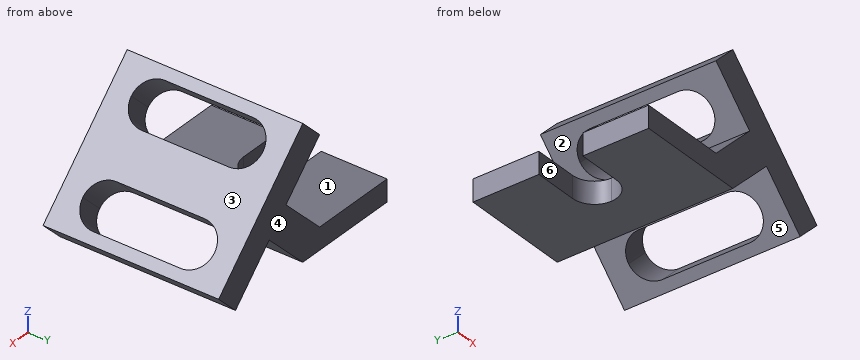
from build123d import *

# Parameters (mm, degrees)
F1_DEPTH = 101.6
F3_DEPTH = 25.4
F5_DEPTH = 37.846


with BuildPart() as f1:
    # F0 (on Front) → F1 (new body, symmetric)
    with BuildSketch(Plane.XZ):
        Polygon((152.4, 76.2), (152.4, 25.4), (177.8, 50.8), (228.6, 0), (254, 25.4), (127, 152.4), (101.6, 127), align=None)
        Polygon((152.4, 76.2), (101.6, 25.4), (152.4, 25.4), align=None)
        Polygon((0, 25.4), (0, 0), (127, 0), (152.4, 25.4), (101.6, 25.4), align=None)
    extrude(amount=F1_DEPTH, both=True)

    # F2 (on face) → F3 (cut)
    with BuildSketch(Plane(origin=(0, 0, 0), x_dir=(1, 0, 0), z_dir=(0, 0, -1))):
        with BuildLine():
            Line((0, 25.4), (0, 0))
            Line((0, 0), (0, -25.4))
            Line((0, -25.4), (50.8, -25.4))
            ThreePointArc((50.8, -25.4), (68.760512, -17.960512), (76.2, 0))
            ThreePointArc((76.2, 0), (68.760512, 17.960512), (50.8, 25.4))
            Line((50.8, 25.4), (0, 25.4))
        make_face()
    extrude(amount=-F3_DEPTH, mode=Mode.SUBTRACT)

    # F4 (on face) → F5 (cut)
    with BuildSketch(Plane(origin=(139.7, 0, 139.7), x_dir=(0, 1, 0), z_dir=(0.707107, 0, 0.707107))):
        with BuildLine():
            ThreePointArc((-76.2, -20.139488), (-68.760512, -38.1), (-50.8, -45.539488))
            Line((-50.8, -45.539488), (50.8, -45.539488))
            ThreePointArc((50.8, -45.539488), (68.760512, -38.1), (76.2, -20.139488))
            ThreePointArc((76.2, -20.139488), (68.760512, -2.178976), (50.8, 5.260512))
            Line((50.8, 5.260512), (-50.8, 5.260512))
            ThreePointArc((-50.8, 5.260512), (-68.760512, -2.178976), (-76.2, -20.139488))
        make_face()
        with BuildLine():
            ThreePointArc((50.8, -148.94461), (68.760512, -141.505122), (76.2, -123.54461))
            ThreePointArc((76.2, -123.54461), (68.760512, -105.584098), (50.8, -98.14461))
            Line((50.8, -98.14461), (-50.8, -98.14461))
            ThreePointArc((-50.8, -98.14461), (-68.760512, -105.584098), (-76.2, -123.54461))
            ThreePointArc((-76.2, -123.54461), (-68.760512, -141.505122), (-50.8, -148.94461))
            Line((-50.8, -148.94461), (50.8, -148.94461))
        make_face()
    extrude(amount=-F5_DEPTH, mode=Mode.SUBTRACT)


solid = f1.part
The model under review builds one solid part; all positions refer to its coordinate system, in mm. Face numbers are marked on the shaded views. A direction names the side the tool comes from. Give positions to 0.01 mm unless a question says otherwise; leave off trailing zeros. Loops run counter-clockwise (first coordinate to the right, second up) from the corner with the lowest first, then second, coordinate; pieces in that order, holes last. Notation, with made-up numbers: (51.25, -17.5) -> (94.25, -17.5) arc R34 cw to (94.25, 21.5) -> close; hole circle Ø3 at (77.5, -15). An arc over 180 degrees is marked (long way). Put each result on its own line as item: value. Start each with the question number.
1. We need section B-B on y = 45. State the section outline as (x, z) points, then the cut area to 3 significant figures.
2. Clearance check with flat-ended pins moving along their axes: P1, Ø3, axis at y = -3.5, z = 118.5, coming from the +X side; P2, Ø10, axis at y = -5, z = 119.5, coming from the -X side; P3, Ø5, axis at y = 5.5, z = 90, coming from the -X side. State where each tip first meets the part, or that it passes through.
3. We need section D-D on y = 3. State the section outline as (x, z) points, then the cut area to 3 significant figures.
4. Wall thickness on probe 1 along Y at (x, z) = (150, 121); probe 2 along Z at (x, y) = (126, 52); probe 3 along Z at (x, y) = (19, 48): over which ranges is each line inside the solid? List them lowest first.
5. Mouldability with a two-part tool opening along Y and no side actions: class the marked faces 4, 5 and 6 as released by +Y, released by -Y, zero draft, split by the parting line, or undercut.
6. We need section C-C on x = 65. State the section outline as (y, z) points, then the cut area to 3 significant figures.
7. We need section A-A on x = 37. State the section outline as (y, z) points, then the cut area to 3 significant figures.
8. For the marked faces 1, 2 and 3, list the 3-axis set-ups (+Z, -Z, +X, -X, +Y, -Y) from which the entire face can be reached by the end or side of a thin tool; tool diameter is ignored.
Determined:
1. outline: (0, 0) -> (127, 0) -> (177.8, 50.8) -> (183.7, 44.9) -> (209.1, 70.3) -> (171.9, 107.5) -> (146.5, 82.1) -> (152.4, 76.2) -> (101.6, 25.4) -> (0, 25.4) -> close; (101.6, 127) -> (110.58, 118.02) -> (135.98, 143.42) -> (127, 152.4) -> close; (219.62, 8.98) -> (228.6, 0) -> (254, 25.4) -> (245.02, 34.38) -> close
1. area: 8,290 mm^2
2. P1: x = 112.56
2. P2: x = 104.1
2. P3: x = 151.9
3. outline: (76.02, 0) -> (127, 0) -> (177.8, 50.8) -> (183.7, 44.9) -> (209.1, 70.3) -> (171.9, 107.5) -> (146.5, 82.1) -> (152.4, 76.2) -> (101.6, 25.4) -> (76.02, 25.4) -> close; (101.6, 127) -> (110.58, 118.02) -> (135.98, 143.42) -> (127, 152.4) -> close; (219.62, 8.98) -> (228.6, 0) -> (254, 25.4) -> (245.02, 34.38) -> close
3. area: 6,350 mm^2
4. probe 1: -101.6 to -76.2, 76.2 to 101.6
4. probe 2: 0 to 49.8, 133.4 to 151.4
4. probe 3: 0 to 25.4
5. face 4: released by +Y
5. face 5: zero draft
5. face 6: undercut
6. outline: (-101.6, 0) -> (-21.06, 0) -> (-21.06, 25.4) -> (-101.6, 25.4) -> close; (21.06, 0) -> (101.6, 0) -> (101.6, 25.4) -> (21.06, 25.4) -> close
6. area: 4,090 mm^2
7. outline: (-101.6, 0) -> (-25.4, 0) -> (-25.4, 25.4) -> (-101.6, 25.4) -> close; (25.4, 0) -> (101.6, 0) -> (101.6, 25.4) -> (25.4, 25.4) -> close
7. area: 3,870 mm^2
8. face 1: +Z, -X, +Y, -Y
8. face 2: -X, +Y, -Y
8. face 3: +Z, +X, +Y, -Y
